Check sheet for the modelled part. Datum: model origin and axes. Units: mm. Give positions to 0.01 mm unless a question says otherwise; leave off trailing zeros. Write each loop counter-clockwise with the first axis right and the second up, starting at its lowest first coordinate (ties: lowest second). Pieces come first, ordered by that corner, then holes. Notation, with made-up numbers: (70.25, 71.25) -> (80.25, 71.25) arc R23 cw to (80.25, 96.25) -> close; hole circle Ø9 at (-28, 3.25). An arc over 180 degrees is marked (long way). Write each question's results on one line, items separated by ' | '. Start each with the question number.
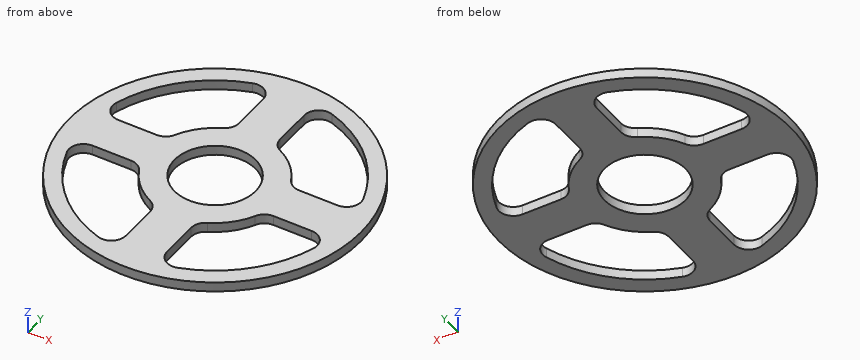
```python
from build123d import *

# Parameters (mm, degrees)
SKETCH_1_R                       = 45
SKETCH_1_R_2                     = 12.5
EXTRUDE_1_DEPTH                  = 1.5
CUT_EXTRUDE_1_DEPTH              = 64.710281745
FILLET_1_R                       = 4.5
PATTERN_CIRCULAR_1_COUNT         = 4
FILLET_1_OF_PATTERN_CIRCULAR_1_R = 4.5


with BuildPart() as part:
    # 스케치1 → 보스-돌출1 (new, symmetric)
    with BuildSketch(Plane.XY):
        Circle(SKETCH_1_R)
        Circle(SKETCH_1_R_2, mode=Mode.SUBTRACT)
    extrude(amount=EXTRUDE_1_DEPTH, both=True)

    # 스케치2 → 컷-돌출1 (cut, through all)
    with BuildSketch(Plane.XY.offset(1.5)):
        with BuildLine():
            Line((6.35, 39.4927525), (6.35, 18.965165436))
            ThreePointArc((6.35, 18.965165436), (14.142135624, 14.142135624), (18.965165436, 6.35))
            Line((18.965165436, 6.35), (39.4927525, 6.35))
            ThreePointArc((39.4927525, 6.35), (28.284271247, 28.284271247), (6.35, 39.4927525))
        make_face()
    cut_extrude_1 = extrude(amount=-CUT_EXTRUDE_1_DEPTH, mode=Mode.SUBTRACT)

    # 필렛1
    fillet_1_edges = [part.edges().sort_by_distance(p)[0] for p in [
        (6.35, 39.4927525, 0),
        (39.4927525, 6.35, 0),
        (18.965165436, 6.35, 0),
        (6.35, 18.965165436, 0),
    ]]
    fillet(fillet_1_edges, radius=FILLET_1_R)

    # 원형 패턴1: 컷-돌출1 ×4 about axis
    pattern_circular_1_axis = Axis((0, 0, 0), (0, 0, 1))
    for i in range(1, PATTERN_CIRCULAR_1_COUNT):
        add(cut_extrude_1.rotate(pattern_circular_1_axis, i * 360 / PATTERN_CIRCULAR_1_COUNT), mode=Mode.SUBTRACT)

    # 필렛1 of 원형 패턴1
    fillet_1_of_pattern_circular_1_edges = [part.edges().sort_by_distance(p)[0] for p in [
        (-39.4927525, 6.35, 0),
        (-6.35, 39.4927525, 0),
        (-6.35, 18.965165436, 0),
        (-18.965165436, 6.35, 0),
        (-6.35, -39.4927525, 0),
        (-39.4927525, -6.35, 0),
        (-18.965165436, -6.35, 0),
        (-6.35, -18.965165436, 0),
        (39.4927525, -6.35, 0),
        (6.35, -39.4927525, 0),
        (6.35, -18.965165436, 0),
        (18.965165436, -6.35, 0),
    ]]
    fillet(fillet_1_of_pattern_circular_1_edges, radius=FILLET_1_OF_PATTERN_CIRCULAR_1_R)


solid = part.part
```
Item 1: Thickness scan on probe 1 along Y at (x, z) = (0, -0.35); probe 2 along Y at (x, z) = (7.5, -1.15); probe 3 along Y at (x, z) = (15.5, 1.15). Record the ranges inside material, lowest first. Write a range as from..to.
Item 2: Section check D-D on z = -1. Count the separate pieces of the cut face and the enclosed holes in it, then the cut area to 3 significant figures.
Item 3: Depth check by flat-ended pin: pin 1 Ø0.9 at (y, z) = (-30.5, -0.5) entering from +X; pin 2 Ø1.5 at (y, z) = (25, 0) entering from +X; pin 3 Ø1.5 at (x, z) = (-30.5, -0.5) entering from -Y. Enter the tip coordinate at first touch or a pass-through.
Item 4: Section check C-C on y = 32.5. Record the boundary of the cut face in (x, z).
Item 5: Section check A-A on x = 0. Record the boundary of the cut face in (y, z), then the cut area to 3 significant figures.
Check sheet entries:
1) probe 1: y = -45..-12.5, 12.5..45 | probe 2: y = -44.37..-36.81, -18.96..-10, 10..18.96, 36.81..44.37 | probe 3: y = -42.25..-36.87, -12.64..12.64, 36.87..42.25
2) separate pieces: 1 | enclosed holes: 5 | area: 3,200 mm^2
3) pin 1: stops at x = 33.5 | pin 2: stops at x = 37.91 | pin 3: stops at y = -33.76
4) outline: (-31.12, -1.5) -> (-23.32, -1.5) -> (-23.32, 1.5) -> (-31.12, 1.5) -> close; (-6.35, -1.5) -> (6.35, -1.5) -> (6.35, 1.5) -> (-6.35, 1.5) -> close; (23.32, -1.5) -> (31.12, -1.5) -> (31.12, 1.5) -> (23.32, 1.5) -> close
5) outline: (-45, -1.5) -> (-12.5, -1.5) -> (-12.5, 1.5) -> (-45, 1.5) -> close; (12.5, -1.5) -> (45, -1.5) -> (45, 1.5) -> (12.5, 1.5) -> close | area: 195 mm^2
